Part model, mm, in its own coordinate system. Face numbers are marked on the shaded views. A direction names the side the tool comes from. Give positions to 0.01 mm unless a question says otherwise; leave off trailing zeros. Order: outer loops, then holes, each group sorted by start corner. A loop starts at its lowest first (then second) coordinate and runs counter-clockwise, first axis right, second up. Notation, with made-up numbers: (45, 6) - (69, 6) arc R22 cw to (69, 41) - close; hole circle Ø4 at (53.25, 62.25). An arc over 180 degrees is marked (long way). One line per item, written item: value.
```python
from build123d import *

# Parameters (mm, degrees)
SKETCH1_W           = 80
SKETCH1_H           = 80
BOSS_EXTRUDE1_DEPTH = 2
SKETCH2_W           = 80
SKETCH2_H           = 80
SKETCH2_W_2         = 78
SKETCH2_H_2         = 78
BOSS_EXTRUDE2_DEPTH = 15
FILLET1_R           = 20
FILLET2_R           = 10
FILLET3_R           = 20
FILLET4_R           = 10
SKETCH3_R           = 1
BOSS_EXTRUDE3_DEPTH = 6
SKETCH4_W           = 10
SKETCH4_H           = 10
BOSS_EXTRUDE4_DEPTH = 5
SKETCH5_W           = 6
SKETCH5_H           = 20
BOSS_EXTRUDE5_DEPTH = 20
CUT_EXTRUDE1_DEPTH  = 23
SKETCH7_R           = 2
CUT_EXTRUDE2_DEPTH  = 23
SKETCH8_R           = 3.5
CUT_EXTRUDE3_DEPTH  = 3
SKETCH9_R           = 1
CUT_EXTRUDE4_DEPTH  = 18
SKETCH10_R          = 1.5
CUT_EXTRUDE5_DEPTH  = 18
SKETCH12_W          = 51.714198926
SKETCH12_H          = 32.805177312
CUT_EXTRUDE7_DEPTH  = 37


with BuildPart() as part:
    # Sketch1 → Boss-Extrude1 (new body)
    with BuildSketch(Plane.XY):
        with Locations((40, 40)):
            Rectangle(SKETCH1_W, SKETCH1_H)
    extrude(amount=BOSS_EXTRUDE1_DEPTH)

    # Sketch2 → Boss-Extrude2 (add)
    with BuildSketch(Plane.XY.offset(2)):
        with Locations((40, 40)):
            Rectangle(SKETCH2_W, SKETCH2_H)
        with Locations((40, 40)):
            Rectangle(SKETCH2_W_2, SKETCH2_H_2, mode=Mode.SUBTRACT)
    extrude(amount=BOSS_EXTRUDE2_DEPTH)

    # Fillet1
    fillet1_edges = [part.edges().sort_by_distance(p)[0] for p in [
        (1, 79, 9.5),
        (1, 1, 9.5),
        (79, 1, 9.5),
        (79, 79, 9.5),
    ]]
    fillet(fillet1_edges, radius=FILLET1_R)

    # Fillet2
    fillet2_edges = [part.edges().sort_by_distance(p)[0] for p in [
        (40, 1, 2),
        (79, 40, 2),
        (40, 79, 2),
        (1, 40, 2),
        (6.857864376, 73.142135624, 2),
        (73.142135624, 73.142135624, 2),
        (6.857864376, 6.857864376, 2),
        (73.142135624, 6.857864376, 2),
    ]]
    fillet(fillet2_edges, radius=FILLET2_R)

    # Fillet3
    fillet3_edges = [part.edges().sort_by_distance(p)[0] for p in [
        (0, 80, 8.5),
        (80, 80, 8.5),
        (80, 0, 8.5),
        (0, 0, 8.5),
    ]]
    fillet(fillet3_edges, radius=FILLET3_R)

    # Fillet4
    fillet4_edges = [part.edges().sort_by_distance(p)[0] for p in [
        (80, 40, 0),
        (0, 40, 0),
        (40, 80, 0),
        (40, 0, 0),
        (5.857864376, 5.857864376, 0),
        (5.857864376, 74.142135624, 0),
        (74.142135624, 74.142135624, 0),
        (74.142135624, 5.857864376, 0),
    ]]
    fillet(fillet4_edges, radius=FILLET4_R)

    # Sketch3 → Boss-Extrude3 (add)
    with BuildSketch(Plane.XY.offset(17)):
        with BuildLine():
            Line((72.292824946, 5.37212195), (70.635028843, 4.105439789))
            Line((70.635028843, 4.105439789), (70.635028843, 7.564971157))
            ThreePointArc((70.635028843, 7.564971157), (71.162236636, 8.837763364), (72.435028843, 9.364971157))
            Line((72.435028843, 9.364971157), (76.003973901, 9.364971157))
            Line((76.003973901, 9.364971157), (72.292824946, 5.37212195))
        make_face()
        with Locations((72.435028843, 7.564971157)):
            Circle(SKETCH3_R, mode=Mode.SUBTRACT)
        with BuildLine():
            Line((9.364971157, 4.105439789), (9.364971157, 7.564971157))
            ThreePointArc((9.364971157, 7.564971157), (8.837763364, 8.837763364), (7.564971157, 9.364971157))
            Line((7.564971157, 9.364971157), (3.996026099, 9.364971157))
            Line((3.996026099, 9.364971157), (7.707175054, 5.37212195))
            Line((7.707175054, 5.37212195), (9.364971157, 4.105439789))
        make_face()
        with Locations((7.564971157, 7.564971157)):
            Circle(SKETCH3_R, mode=Mode.SUBTRACT)
        with BuildLine():
            Line((70.635028843, 75.894560211), (70.635028843, 72.435028843))
            ThreePointArc((70.635028843, 72.435028843), (71.162236636, 71.162236636), (72.435028843, 70.635028843))
            Line((72.435028843, 70.635028843), (76.003973901, 70.635028843))
            Line((76.003973901, 70.635028843), (72.292824946, 74.62787805))
            Line((72.292824946, 74.62787805), (70.635028843, 75.894560211))
        make_face()
        with Locations((72.435028843, 72.435028843)):
            Circle(SKETCH3_R, mode=Mode.SUBTRACT)
        with BuildLine():
            Line((7.707175054, 74.62787805), (9.364971157, 75.894560211))
            Line((9.364971157, 75.894560211), (9.364971157, 72.435028843))
            ThreePointArc((9.364971157, 72.435028843), (8.837763364, 71.162236636), (7.564971157, 70.635028843))
            Line((7.564971157, 70.635028843), (3.996026099, 70.635028843))
            Line((3.996026099, 70.635028843), (7.707175054, 74.62787805))
        make_face()
        with Locations((7.564971157, 72.435028843)):
            Circle(SKETCH3_R, mode=Mode.SUBTRACT)
    extrude(amount=-BOSS_EXTRUDE3_DEPTH)

    # Sketch4 → Boss-Extrude4 (add)
    with BuildSketch(Plane(origin=(0, 0, 0), x_dir=(-1, 0, 0), z_dir=(0, 0, -1))):
        with Locations((-35, 35)):
            Rectangle(SKETCH4_W, SKETCH4_H)
        with Locations((-35, 45)):
            Rectangle(SKETCH4_W, SKETCH4_H)
        with Locations((-45, 45)):
            Rectangle(SKETCH4_W, SKETCH4_H)
        with Locations((-45, 35)):
            Rectangle(SKETCH4_W, SKETCH4_H)
    extrude(amount=BOSS_EXTRUDE4_DEPTH)

    # Sketch5 → Boss-Extrude5 (add)
    with BuildSketch(Plane(origin=(0, 0, -5), x_dir=(-1, 0, 0), z_dir=(0, 0, -1))):
        with Locations((-33, 40)):
            Rectangle(SKETCH5_W, SKETCH5_H)
        with Locations((-47, 40)):
            Rectangle(SKETCH5_W, SKETCH5_H)
    extrude(amount=BOSS_EXTRUDE5_DEPTH)

    # Sketch6 → Cut-Extrude1 (cut)
    with BuildSketch(Plane.ZY.offset(-30)):
        with BuildLine():
            Line((-15, 30), (-19.756708154, 21.186247086))
            Line((-19.756708154, 21.186247086), (-29.168380108, 27.64799201))
            Line((-29.168380108, 27.64799201), (-29.168380108, 53.846153493))
            Line((-29.168380108, 53.846153493), (-15, 50))
            ThreePointArc((-15, 50), (-25, 40), (-15, 30))
        make_face()
    extrude(amount=-CUT_EXTRUDE1_DEPTH, mode=Mode.SUBTRACT)

    # Sketch7 → Cut-Extrude2 (cut)
    with BuildSketch(Plane.ZY.offset(-30)):
        with Locations((-15, 40)):
            Circle(SKETCH7_R)
    extrude(amount=-CUT_EXTRUDE2_DEPTH, mode=Mode.SUBTRACT)

    # Sketch8 → Cut-Extrude3 (cut)
    with BuildSketch(Plane.ZY.offset(-30)):
        with Locations((-15, 40)):
            Circle(SKETCH8_R)
    extrude(amount=-CUT_EXTRUDE3_DEPTH, mode=Mode.SUBTRACT)

    # Sketch9 → Cut-Extrude4 (cut)
    with BuildSketch(Plane(origin=(0, 0, -5), x_dir=(-1, 0, 0), z_dir=(0, 0, -1))):
        with Locations((-40, 45)):
            Circle(SKETCH9_R)
        with Locations((-40, 35)):
            Circle(SKETCH9_R)
    extrude(amount=-CUT_EXTRUDE4_DEPTH, mode=Mode.SUBTRACT)

    # Sketch10 → Cut-Extrude5 (cut)
    with BuildSketch(Plane(origin=(0, 0, -5), x_dir=(-1, 0, 0), z_dir=(0, 0, -1))):
        with Locations((-40, 40)):
            Circle(SKETCH10_R)
    extrude(amount=-CUT_EXTRUDE5_DEPTH, mode=Mode.SUBTRACT)

    # Sketch12 → Cut-Extrude7 (cut)
    with BuildSketch(Plane.XZ.offset(-30)):
        with Locations((40.307091443, -16.402588656)):
            Rectangle(SKETCH12_W, SKETCH12_H)
    extrude(amount=-CUT_EXTRUDE7_DEPTH, mode=Mode.SUBTRACT)


solid = part.part
```
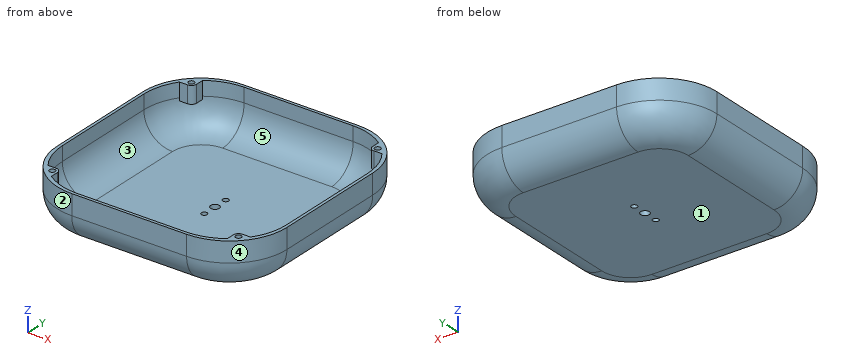
1) Which spindle directions (+Z, -Z, +X, -X, +Y, -Y) get a long thin tool onto all of the face, cutting with end or side? Do the marked faces 4 and 5. Say none if no direction does.
Answer:
face 4: +Z, -Z, +X, -Y
face 5: +Z
2) Two-plate mould, pull along X, no slides. Class the marked faces 1, 2 and 3: pulls with the +X half, pulls with the -X half, needs draft (parallel to the pull), parting line crosses it, or undercut.
Answer:
face 1: needs draft
face 2: pulls with the -X half
face 3: undercut
3) Wall check: line 1 along X through (y, z) = (46.5, 15.25); line 2 along Y through (x, z) = (40, 1.3); line 3 along Y through (x, z) = (40, 1.25). Give the ranges that are in metal, low to high. Write a range as [from, to].
Answer:
line 1: x = [0, 1], [79, 80]
line 2: y = [5.07, 34], [36, 38.5], [41.5, 44], [46, 74.93]
line 3: y = [5.16, 34], [36, 38.5], [41.5, 44], [46, 74.84]
4) Slice it at C-C on y = 51. Write the cut outline in (x, z), then the cut area to 3 significant figures.
Answer:
outline: (0, 10) arc R10 ccw to (10, 0) - (70, 0) arc R10 ccw to (80, 10) - (80, 17) - (79, 17) - (79, 12) arc R10 cw to (69, 2) - (11, 2) arc R10 cw to (1, 12) - (1, 17) - (0, 17) - close
area: 190 mm2
5) Slice it at A-A on y = 35. Write the cut outline in (x, z), then the cut area to 3 significant figures.
Answer:
outline: (0, 10) arc R10 ccw to (10, 0) - (39, 0) - (39, 2) - (11, 2) arc R10 cw to (1, 12) - (1, 17) - (0, 17) - close; (41, 0) - (70, 0) arc R10 ccw to (80, 10) - (80, 17) - (79, 17) - (79, 12) arc R10 cw to (69, 2) - (41, 2) - close
area: 186 mm2
6) Drop flat-ended pins along their axis: P1, Ø5, axis at x = 10, z = 4, coming from the +Y side; P2, Ø2.5, axis at y = 6, z = 14.5, coming from the -X side; P3, Ø2, axis at x = 47.5, z = 6.5, coming from the +Y side. Give the stop position or say it passes through.
Answer:
P1: stops at y = 77.19
P2: stops at x = 4.59
P3: stops at y = 79.68
7) Slice it at D-D on z = 13.5. Count the separate pieces of the cut face and the enclosed holes in it, then the cut area to 3 significant figures.
Answer:
separate pieces: 1
enclosed holes: 5
area: 348 mm2
8) Slice it at B-B on x = 40. Write the cut outline in (y, z).
Answer:
outline: (0, 10) arc R10 ccw to (10, 0) - (34, 0) - (34, 2) - (11, 2) arc R10 cw to (1, 12) - (1, 17) - (0, 17) - close; (36, 0) - (38.5, 0) - (38.5, 2) - (36, 2) - close; (41.5, 0) - (44, 0) - (44, 2) - (41.5, 2) - close; (46, 0) - (70, 0) arc R10 ccw to (80, 10) - (80, 17) - (79, 17) - (79, 12) arc R10 cw to (69, 2) - (46, 2) - close
